Check sheet for the modelled part. Datum: model origin and axes. Units: mm. Face numbers are marked on the shaded views. A direction names the side the tool comes from. Give positions to 0.01 mm unless a question says otherwise; leave off trailing zeros. Order: outer loops, then holes, each group sorted by start corner. A loop starts at its lowest first (then second) coordinate and runs counter-clockwise, first axis right, second up.
from build123d import *

# Parameters (mm, degrees)
ESQUISSE1_W             = 34
ESQUISSE1_H             = 5
BOSS_EXTRU_1_DEPTH      = 20
ESQUISSE2_R             = 4.5
ENL_V_MAT_EXTRU_1_DEPTH = 5
ESQUISSE5_W             = 20
ESQUISSE5_H             = 5
BOSS_EXTRU_2_DEPTH      = 80
ESQUISSE6_R             = 2.5
ENL_V_MAT_EXTRU_2_DEPTH = 5


with BuildPart() as part:
    # Esquisse1 → Boss.-Extru.1 (new body)
    with BuildSketch(Plane.XY):
        Polygon((-21.374377126, 20.152588272), (-21.374377126, 25.152588272), (-26.374377126, 25.152588272), (-26.374377126, -34.847411728), (-21.374377126, -34.847411728), align=None)
        with Locations((-4.374377126, 22.652588272)):
            Rectangle(ESQUISSE1_W, ESQUISSE1_H)
        Polygon((17.625622874, 25.152588272), (12.625622874, 25.152588272), (12.625622874, 20.152588272), (12.625622874, 10.152588272), (17.625622874, 10.152588272), align=None)
        Polygon((12.625622874, -34.847411728), (-21.374377126, -34.847411728), (-26.374377126, -34.847411728), (-26.374377126, -39.847411728), (12.625622874, -39.847411728), align=None)
    extrude(amount=BOSS_EXTRU_1_DEPTH)

    # Esquisse2 → Enlèv. mat.-Extru.1 (cut)
    with BuildSketch(Plane.XZ.offset(39.847411728)):
        with Locations((-4.219859272, 10)):
            Circle(ESQUISSE2_R)
    extrude(amount=-ENL_V_MAT_EXTRU_1_DEPTH, mode=Mode.SUBTRACT)

    # Esquisse5 → Boss.-Extru.2 (add)
    with BuildSketch(Plane(origin=(12.625622874, 0, 0), x_dir=(0, 0, -1), z_dir=(1, 0, 0))):
        with Locations((-10, -37.347411728)):
            Rectangle(ESQUISSE5_W, ESQUISSE5_H)
    extrude(amount=BOSS_EXTRU_2_DEPTH)

    # Esquisse6 → Enlèv. mat.-Extru.2 (cut)
    with BuildSketch(Plane.XZ.offset(39.847411728)):
        with Locations((82.625622874, 10)):
            Circle(ESQUISSE6_R)
        with Locations((72.625622874, 10)):
            Circle(ESQUISSE6_R)
        with Locations((62.625622874, 10)):
            Circle(ESQUISSE6_R)
        with Locations((52.625622874, 10)):
            Circle(ESQUISSE6_R)
        with Locations((42.625622874, 10)):
            Circle(ESQUISSE6_R)
    extrude(amount=-ENL_V_MAT_EXTRU_2_DEPTH, mode=Mode.SUBTRACT)


solid = part.part
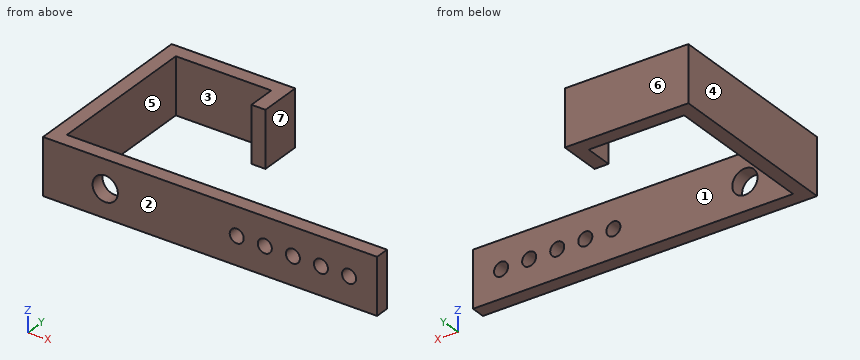
1) Section check D-D, the plane z = 18.25. Record the cut outline in (x, y), then the cut area to 3 significant figures.
Recorded:
outline: (-26.37, -39.85) - (92.63, -39.85) - (92.63, -34.85) - (-21.37, -34.85) - (-21.37, 20.15) - (12.63, 20.15) - (12.63, 10.15) - (17.63, 10.15) - (17.63, 25.15) - (-26.37, 25.15) - close
area: 1,140 mm2
2) Section check B-B, the plane y = 11.5. Record the cut outline in (x, z).
Recorded:
outline: (-26.37, 0) - (-21.37, 0) - (-21.37, 20) - (-26.37, 20) - close; (12.63, 0) - (17.63, 0) - (17.63, 20) - (12.63, 20) - close
3) Depth check by flat-ended pin: pin 1 Ø5 at (x, z) = (38.5, 13) entering from +Y; pin 2 Ø5 at (y, z) = (5, 3) entering from +X; pin 3 Ø4.5 at (x, z) = (72.63, 10) entering from +Y; pin 4 Ø7 at (x, z) = (-4.22, 10) entering from -Y. Enter the tip coordinate at first touch or a pass-through.
Recorded:
pin 1: stops at y = -34.85
pin 2: stops at x = -21.37
pin 3: passes through
pin 4: stops at y = 20.15
4) Set-up check for the marked faces 1, 2 and 3: record each of +Z, -Z, +X, -X, +Y, -Y from which the full face is reachable in a straight line by a thin tool's end or side.
Recorded:
face 1: +Z, -Z, +X
face 2: +Z, -Z, +X, -X, -Y
face 3: +Z, -Z
5) Material ranges on L1, parallel to Y at x = 17.5, z = 5.25; L2, parallel to Y at x = 12, z = 6.75; L3, parallel to X at y = 14, z = 8, recorded low to high.
Recorded:
L1: y = -39.85 to -34.85, 10.15 to 25.15
L2: y = -39.85 to -34.85, 20.15 to 25.15
L3: x = -26.37 to -21.37, 12.63 to 17.63
6) Draft check along X on the marked faces 4, 5, 6 and 7. Enter one of: +X half, -X half, draft (parallel to the pull), parting line (faces both ways), or undercut.
Recorded:
face 4: -X half
face 5: undercut
face 6: draft
face 7: +X half
7) Section check C-C, the plane x = 6. Record the cut outline in (y, z), then the cut area to 3 significant figures.
Recorded:
outline: (-39.85, 0) - (-34.85, 0) - (-34.85, 20) - (-39.85, 20) - close; (20.15, 0) - (25.15, 0) - (25.15, 20) - (20.15, 20) - close
area: 200 mm2
8) Section check A-A, the plane z = 10. State how many separate pieces and enclosed holes the cut face has, then the cut area to 3 significant figures.
Recorded:
separate pieces: 7
enclosed holes: 0
area: 970 mm2
